from build123d import *

# Parameters (mm, degrees)
SKETCH1_R               = 35
BOSS_EXTRUDE1_DEPTH     = 11
BOSS_EXTRUDE2_START     = 8
SKETCH2_W               = 9.919125271
SKETCH2_H               = 19.24261003
BOSS_EXTRUDE2_DEPTH     = 8
SKETCH4_W               = 19.49756264
SKETCH4_H               = 18.874094786
BOSS_EXTRUDE3_DEPTH     = 8
SKETCH6_R               = 5.918890508
CUT_EXTRUDE1_DEPTH      = 5
CUT_EXTRUDE4_DEPTH      = 16
CUT_EXTRUDE4_DEPTH_BACK = 5


with BuildPart() as part:
    # Sketch1 → Boss-Extrude1 (new body)
    with BuildSketch(Plane.XY):
        Circle(SKETCH1_R)
    extrude(amount=BOSS_EXTRUDE1_DEPTH)

    # Sketch2 → Boss-Extrude2 (add)
    with BuildSketch(Plane(origin=(0, 0, 0), x_dir=(-1, 0, 0), z_dir=(0, 0, -1)).offset(BOSS_EXTRUDE2_START)):
        with BuildLine():
            Line((-18.0511494, 9.437047393), (-31.70374069, 9.437047393))
            ThreePointArc((-31.70374069, 9.437047393), (-33.117954252, 8.851260956), (-33.70374069, 7.437047393))
            Line((-33.70374069, 7.437047393), (-33.70374069, 4.679927622))
            Line((-33.70374069, 4.679927622), (-29.859553671, 4.679927622))
            ThreePointArc((-29.859553671, 4.679927622), (-29.15244689, 4.387034403), (-28.859553671, 3.679927622))
            Line((-28.859553671, 3.679927622), (-28.859553671, 0))
            Line((-28.859553671, 0), (-28.859553671, -3.679927622))
            ThreePointArc((-28.859553671, -3.679927622), (-29.15244689, -4.387034403), (-29.859553671, -4.679927622))
            Line((-29.859553671, -4.679927622), (-33.70374069, -4.679927622))
            Line((-33.70374069, -4.679927622), (-33.70374069, -7.582708941))
            ThreePointArc((-33.70374069, -7.582708941), (-33.117954252, -8.996922503), (-31.70374069, -9.582708941))
            Line((-31.70374069, -9.582708941), (-18.0511494, -9.582708941))
            Line((-18.0511494, -9.582708941), (-18.0511494, -9.437047393))
            ThreePointArc((-18.0511494, -9.437047393), (-10.791286921, -16.696909873), (-18.0511494, -23.956772352))
            Line((-18.0511494, -23.956772352), (-18.0511494, -28.833324521))
            ThreePointArc((-18.0511494, -28.833324521), (-17.775329476, -29.846834791), (-17.023946334, -30.580798734))
            ThreePointArc((-17.023946334, -30.580798734), (-14.809870149, -31.712264917), (-12.521051282, -32.683685147))
            ThreePointArc((-12.521051282, -32.683685147), (-10.672199785, -32.463919973), (-9.805562637, -30.816045996))
            Line((-9.805562637, -30.816045996), (-9.805562637, 9.437047393))
            Line((-9.805562637, 9.437047393), (-9.805562637, 30.816045996))
            ThreePointArc((-9.805562637, 30.816045996), (-10.672199785, 32.463919973), (-12.521051282, 32.683685147))
            ThreePointArc((-12.521051282, 32.683685147), (-14.809870149, 31.712264917), (-17.023946334, 30.580798734))
            ThreePointArc((-17.023946334, 30.580798734), (-17.775329476, 29.84683479), (-18.0511494, 28.833324521))
            Line((-18.0511494, 28.833324521), (-18.0511494, 23.956772352))
            ThreePointArc((-18.0511494, 23.956772352), (-10.791286921, 16.696909873), (-18.0511494, 9.437047393))
        make_face()
        with BuildLine():
            ThreePointArc((32.652182779, 6.91093898), (24.692534845, 23.296158989), (9.692000003, 33.631311838))
            Line((9.692000003, 33.631311838), (9.692000003, 9.437047393))
            Line((9.692000003, 9.437047393), (19.611125274, 9.437047393))
            Line((19.611125274, 9.437047393), (19.611125274, -9.805562637))
            Line((19.611125274, -9.805562637), (9.692000003, -9.805562637))
            Line((9.692000003, -9.805562637), (9.692000003, -33.631311838))
            ThreePointArc((9.692000003, -33.631311838), (24.692534845, -23.296158989), (32.652182779, -6.91093898))
            ThreePointArc((32.652182779, -6.91093898), (32.443493864, -6.082517787), (31.671050481, -5.717601419))
            Line((31.671050481, -5.717601419), (27.071040834, -5.717601419))
            ThreePointArc((27.071040834, -5.717601419), (25.656827271, -5.131814981), (25.071040834, -3.717601419))
            Line((25.071040834, -3.717601419), (25.071040834, 3.717601419))
            ThreePointArc((25.071040834, 3.717601419), (25.656827271, 5.131814981), (27.071040834, 5.717601419))
            Line((27.071040834, 5.717601419), (31.671050481, 5.717601419))
            ThreePointArc((31.671050481, 5.717601419), (32.443493864, 6.082517787), (32.652182779, 6.91093898))
        make_face()
        with Locations((14.651562639, -0.184257622)):
            Rectangle(SKETCH2_W, SKETCH2_H)
    extrude(amount=-BOSS_EXTRUDE2_DEPTH)

    # Sketch4 → Boss-Extrude3 (add)
    with BuildSketch(Plane(origin=(0, 0, 0), x_dir=(-1, 0, 0), z_dir=(0, 0, -1))):
        with Locations((-0.056781317, 0)):
            Rectangle(SKETCH4_W, SKETCH4_H)
    extrude(amount=BOSS_EXTRUDE3_DEPTH)

    # Sketch6 → Cut-Extrude1 (cut)
    with BuildSketch(Plane(origin=(0, 0, -8), x_dir=(-1, 0, 0), z_dir=(0, 0, -1))):
        with Locations((18.756852772, 16.696909873)):
            Circle(SKETCH6_R)
        with Locations(Location((18.756852772, -16.696909873, 0), (0, 0, 180))):
            Circle(SKETCH6_R)
    extrude(amount=-CUT_EXTRUDE1_DEPTH, mode=Mode.SUBTRACT)

    # Sketch11 → Cut-Extrude4 (cut, two sides: drawn at the far end of the back side and taken through both)
    with BuildSketch(Plane(origin=(0, 4.679927622, 0), x_dir=(-1, 0, 0), z_dir=(0, -1, 0)).offset(-CUT_EXTRUDE4_DEPTH_BACK)):
        with BuildLine():
            Line((-33.70374069, 6.745944891), (-33.70374069, 1.4705717))
            ThreePointArc((-33.70374069, 1.4705717), (-33.58881267, 1.789506757), (-33.296862408, 1.961823515))
            ThreePointArc((-33.296862408, 1.961823515), (-31.519082318, 4.108258295), (-33.296862408, 6.254693076))
            ThreePointArc((-33.296862408, 6.254693076), (-33.58881267, 6.427009834), (-33.70374069, 6.745944891))
        make_face()
    extrude(amount=CUT_EXTRUDE4_DEPTH + CUT_EXTRUDE4_DEPTH_BACK, mode=Mode.SUBTRACT)


solid = part.part
Source: CAD feature listing. Evaluate the final solid. Frame: model axes, mm. A direction names the side the tool comes from. Give positions to 0.01 mm unless a question says otherwise; leave off trailing zeros. Order: outer loops, then holes, each group sorted by start corner. A loop starts at its lowest first (then second) coordinate and runs counter-clockwise, first axis right, second up. Notation, with made-up numbers: (38.25, 6) -> (80.25, 6) arc R20 cw to (80.25, 29) -> close; hole circle Ø1 at (86.5, -28). An arc over 180 degrees is marked (long way). Write item = value, one per line.
Q1. Pull-direction query (Z, two-part tool) for faces 4 (the face through (1, 0, -8)), 5 (the face through (31.52, -7.1, -4.07)), 6 (the face through (9.806, 20, -4)); classes: released by +Z, released by -Z, zero draft, split by the parting line, or undercut.
Data:
face_4 = released by -Z
face_5 = undercut
face_6 = zero draft
Q2. Set-up query: faces 1 (the face through (-24.524, -23.491, -4.056)), 2 (the face through (28.86, 0, -4)), 3 (the face through (-24.86, 23.1, -4.06)). Return all of +Z, -Z, +X, -X, +Y, -Y with unobstructed straight access to the full face (end or side cutting, diameter ignored); none if empty.
Data:
face_1 = -Z, -X, -Y
face_2 = -Z, +X
face_3 = -Z, -X, +Y
Q3. Pin query (flat end, axial travel): pin 1 (1 mm diameter, centred on x = -18, y = -18.5, fed in from -Z); pin 2 (1 mm diameter, centred on x = 10, z = 2, fed in from -Y); pin 3 (4 mm diameter, centred on y = -15.5, z = -4, fed in from +X). Return the tip coordinate at first contact, or that it passes through.
Data:
pin_1 = -3
pin_2 = -33.69
pin_3 = 11.53
Q4. Cut plane B-B, the plane y = 0. Output: boundary loops of the cut face in (x, z).
Data:
outline = (-35, 0) -> (-25.07, 0) -> (-25.07, -8) -> (28.86, -8) -> (28.86, 0) -> (35, 0) -> (35, 11) -> (-35, 11) -> close
Q5. Cut plane A-A, the plane x = 21. Output: boundary loops of the cut face in (y, z).
Data:
outline = (-28, 0) -> (-9.58, 0) -> (-9.58, -8) -> (9.44, -8) -> (9.44, 0) -> (28, 0) -> (28, 11) -> (-28, 11) -> close
Q6. Material intervals for line 1 (X direction, y = -21, z = -4.5); line 2 (Y direction, x = 15.5, z = -3.5); line 3 (Z direction, x = 2, y = 23.5), sorted ascending. Write a range as from..to.
Data:
line_1 = -26.51..-22.82, -14.69..-9.69, 9.81..12.2
line_2 = -31.38..-23.49, -9.9..9.9, 23.49..31.38
line_3 = 0..11
Q7. Cut plane C-C, the plane z = 9. Output: boundary loops of the cut face in (x, y).
Data:
outline = circle Ø70 at (0, 0)
Q8. Cut plane D-D, the plane x = -22. Output: boundary loops of the cut face in (y, z), and give its area (3 significant figures).
Data:
outline = (-27.22, 0) -> (-26.1, 0) -> (-26.1, -8) -> (-21.65, -8) -> (-21.65, -3) -> (-11.75, -3) -> (-11.75, -8) -> (11.75, -8) -> (11.75, -3) -> (21.65, -3) -> (21.65, -8) -> (26.1, -8) -> (26.1, 0) -> (27.22, 0) -> (27.22, 11) -> (-27.22, 11) -> close
area = 918 mm^2
